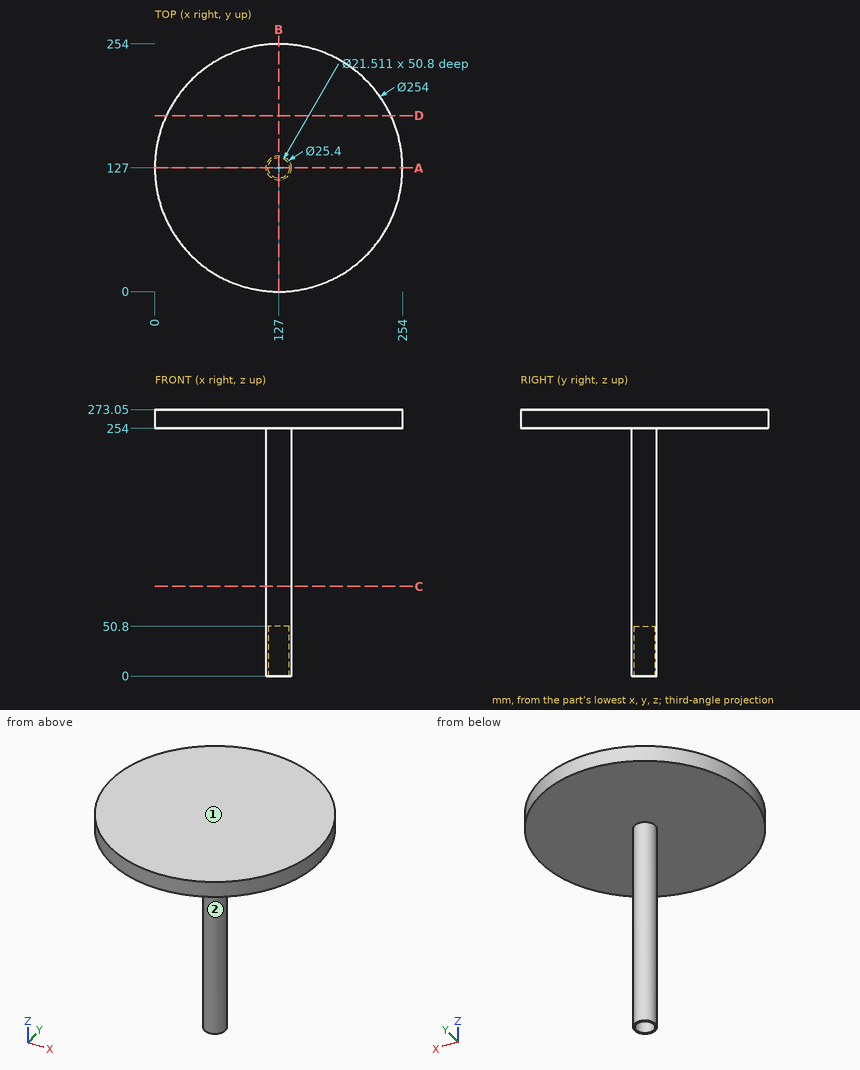
Print and shaded views of the part. All mm, measured from the part's lowest x, y and z. A direction names the side the tool comes from. Round coordinates to 2 decimals unless told otherwise and drop trailing zeros. Write each loop counter-clockwise with the first axis right and the second up, starting at its lowest first coordinate (ties: lowest second). Pieces come first, ordered by that corner, then holes.
Item 1: Which spindle directions (+Z, -Z, +X, -X, +Y, -Y) get a long thin tool onto all of the face, cutting with end or side? Do the marked faces 1 and 2. Say none if no direction does.
Results:
face 1: +Z, +X, -X, +Y, -Y
face 2: -Z
Item 2: Cut at C-C, the plane z = 92. Give the cut face in (x, y).
Results:
outline: circle Ø25.4 at (127, 127)
Item 3: Cut at D-D, the plane y = 180.5. Give the cut face in (x, z), plus the area to 3 significant figures.
Results:
outline: (11.82, 254) - (242.18, 254) - (242.18, 273.05) - (11.82, 273.05) - close
area: 4,390 mm2
Item 4: Probe L1, parallel to X at y = 127, z = 17; L2, parallel to Z at x = 103, y = 57. List the from-to ranges inside material, lowest first.
Results:
L1: x = 114.3 to 116.24, 137.76 to 139.7
L2: z = 254 to 273.05
Item 5: Drop flat-ended pins along their axis: pin 1 Ø10 at (x, z) = (145, 233.5) entering from -Y; pin 2 Ø17 at (x, y) = (128.5, 126.5) entering from -Z. Give the stop position or say it passes through.
Results:
pin 1: passes through
pin 2: stops at z = 50.8
Item 6: Cut at A-A, the plane y = 127. Give the cut face in (x, z).
Results:
outline: (0, 254) - (114.3, 254) - (114.3, 0) - (116.24, 0) - (116.24, 50.8) - (137.76, 50.8) - (137.76, 0) - (139.7, 0) - (139.7, 254) - (254, 254) - (254, 273.05) - (0, 273.05) - close
